from build123d import *

# Parameters (mm, degrees)
SKETCH1_W           = 50
SKETCH1_H           = 35
BOSS_EXTRUDE1_DEPTH = 12
BOSS_EXTRUDE2_DEPTH = 2
FILLET1_R           = 2
SKETCH4_R           = 1.39
CUT_EXTRUDE1_DEPTH  = 34.574543928


with BuildPart() as part:
    # Sketch1 → Boss-Extrude1 (new body)
    with BuildSketch(Plane(origin=(0, 0, 0), x_dir=(1, 0, 0), z_dir=(0, 1, 0))):
        Rectangle(SKETCH1_W, SKETCH1_H)
    extrude(amount=BOSS_EXTRUDE1_DEPTH)

    # Sketch2 → Boss-Extrude2 (add)
    with BuildSketch(Plane(origin=(0, 12, 0), x_dir=(1, 0, 0), z_dir=(0, 1, 0))):
        with BuildLine():
            Line((-8, 10), (-8, 5))
            ThreePointArc((-8, 5), (-10, 3), (-12, 5))
            Line((-12, 5), (-12, 10))
            ThreePointArc((-12, 10), (-10, 12), (-8, 10))
        make_face()
        with BuildLine():
            Line((-8, -5), (-8, -10))
            ThreePointArc((-8, -10), (-10, -12), (-12, -10))
            Line((-12, -10), (-12, -5))
            ThreePointArc((-12, -5), (-10, -3), (-8, -5))
        make_face()
    extrude(amount=BOSS_EXTRUDE2_DEPTH)

    # Fillet1
    fillet1_edges = [part.edges().sort_by_distance(p)[0] for p in [
        (-25, 12, 0),
        (0, 12, 17.5),
        (25, 12, 0),
        (0, 12, -17.5),
        (25, 6, 17.5),
        (-25, 6, 17.5),
        (-25, 6, -17.5),
        (25, 6, -17.5),
    ]]
    fillet(fillet1_edges, radius=FILLET1_R)

    # Sketch4 → Cut-Extrude1 (cut, through all)
    with BuildSketch(Plane.XZ):
        with Locations(Location((-19.5, 12, 0), (0, 0, 270))):
            Circle(SKETCH4_R)
        with Locations(Location((19.5, -12, 0), (0, 0, 270))):
            Circle(SKETCH4_R)
    extrude(amount=-CUT_EXTRUDE1_DEPTH, mode=Mode.SUBTRACT)


solid = part.part
Here's how the part is built. I have some questions about the finished solid (model axes, mm). A direction names the side the tool comes from. Give positions to 0.01 mm unless a question says otherwise; leave off trailing zeros. Loops run counter-clockwise (first coordinate to the right, second up) from the corner with the lowest first, then second, coordinate; pieces in that order, holes last. Notation, with made-up numbers: (-29.75, -37) -> (29.25, -37) arc R32 ccw to (29.25, -8) -> close; hole circle Ø10 at (8.5, 55). An arc over 180 degrees is marked (long way). Answer as a JSON object with one key per item and string values. Group by question number.
Item 1: Will these pins go through, and if not, where does the flat tip stop? pin 1 (1 mm diameter, centred on y = 13, z = 8.5, fed in from -X); pin 2 (1.6 mm diameter, centred on y = 12.5, z = -8, fed in from +X); pin 3 (15.5 mm diameter, centred on x = 0.5, z = -7.5, fed in from +Y); pin 4 (1.7 mm diameter, centred on x = -19.5, z = 12, fed in from -Y).
Item 2: Imagine slicing it at A-A on x = 19.5. Write out the boundary of the cut face in (y, z).
Item 3: Imagine slicing it at C-C on z = -2. Write out the boundary of the cut face in (x, y), then the cut area to 3 significant figures.
Item 4: On a 3-axis mill with a long thin cutter (end or side, diameter ignored), from which of +Z, -Z, +X, -X, +Y, -Y can I reach the whole of each face in a straight line? I mean faces 1 (the flat face through (-10, 14, 7)), 2 (the flat face through (-8, 13, -8)), 3 (the cylindrical face through (-10, 13, 3)), 4 (the flat face through (-12, 13, -7)), 5 (the cylindrical face through (-24.43, 5.07, -16.9)). Say none if no direction works.
Item 5: Imagine slicing it at B-B on x = 10.5. Write out the boundary of the cut face in (y, z).
Item 6: I need wall thicknesses on L1, parallel to X at y = 9, z = -12; L2, parallel to X at y = 7.5, z = 12; L3, parallel to Y at x = 17, z = -15. Which ranges of each line are inside material? Lowest first, please.
Answer list:
{
 "1": {"pin 1": "stops at x = -12", "pin 2": "stops at x = 24.05", "pin 3": "stops at y = 12", "pin 4": "passes through"},
 "2": {"outline": "(0, -17.5) -> (10, -17.5) arc R2 ccw to (12, -15.5) -> (12, -13.39) -> (0, -13.39) -> close; (0, -10.61) -> (12, -10.61) -> (12, 15.5) arc R2 ccw to (10, 17.5) -> (0, 17.5) -> close"},
 "3": {"outline": "(-25, 0) -> (25, 0) -> (25, 10) arc R2 ccw to (23, 12) -> (-23, 12) arc R2 ccw to (-25, 10) -> close", "area": "598 mm2"},
 "4": {"face 1": "+Z, -Z, +X, -X, +Y", "face 2": "+Z, -Z, +X, +Y", "face 3": "+Y", "face 4": "+Z, -Z, -X, +Y", "face 5": "-Z, -X, +Y, -Y"},
 "5": {"outline": "(0, -17.5) -> (10, -17.5) arc R2 ccw to (12, -15.5) -> (12, 15.5) arc R2 ccw to (10, 17.5) -> (0, 17.5) -> close"},
 "6": {"L1": "x = -25 to 18.11, 20.89 to 25", "L2": "x = -25 to -20.89, -18.11 to 25", "L3": "y = 0 to 12"}
}
